```python
from build123d import *

# Parameters (mm, degrees)
CROQUIS1_W                 = 115
CROQUIS1_H                 = 76
SALIENTE_EXTRUIR1_DEPTH    = 1.5
CORTAR_EXTRUIR2_DEPTH      = 2.5
MATRIZL4_COUNT             = 3
MATRIZL4_PITCH             = 38.333333333
SIMETR_A1_COPY_1_DEPTH     = 2.5
SIMETR_A1_COPY_2_DEPTH     = 2.5
CORTAR_EXTRUIR3_DEPTH      = 2.5
MATRIZL5_COUNT             = 2
MATRIZL5_PITCH             = 38
SIMETR_A2_COPY_1_DEPTH     = 2.5
CROQUIS2_R                 = 1.2
CORTAR_EXTRUIR1_DEPTH      = 2.5
CORTAR_EXTRUIR1_DEPTH_BACK = 2.5
CROQUIS5_W                 = 9.5
CROQUIS5_H                 = 3
CROQUIS5_W_2               = 19
SALIENTE_EXTRUIR2_DEPTH    = 17
CROQUIS6_W                 = 19
CROQUIS6_H                 = 3
SALIENTE_EXTRUIR3_DEPTH    = 17


with BuildPart() as part:
    # Croquis1 → Saliente-Extruir1 (new body, symmetric)
    with BuildSketch(Plane(origin=(0, 0, 0), x_dir=(1, 0, 0), z_dir=(0, 1, 0))):
        Rectangle(CROQUIS1_W, CROQUIS1_H)
    extrude(amount=SALIENTE_EXTRUIR1_DEPTH, both=True)

    # Croquis3 → Cortar-Extruir2 (cut, symmetric)
    with BuildSketch(Plane(origin=(0, 0, 0), x_dir=(1, 0, 0), z_dir=(0, 1, 0))):
        Polygon((-47.916666667, -35), (-39.483333333, -35), (-37.183333333, -35), (-28.75, -35), (-28.75, -38), (-47.916666667, -38), align=None)
    cortar_extruir2 = extrude(amount=CORTAR_EXTRUIR2_DEPTH, both=True, mode=Mode.SUBTRACT)

    # MatrizL4: Cortar-Extruir2 ×3
    with Locations(*[(i * MATRIZL4_PITCH, 0, 0) for i in range(1, MATRIZL4_COUNT)]):
        add(cortar_extruir2, mode=Mode.SUBTRACT)

    # Simetría1: Cortar-Extruir2 across plane
    add(cortar_extruir2.mirror(Plane.XY), mode=Mode.SUBTRACT)

    # Simetría1 copy 1 sketch → Simetría1 copy 1 (cut, symmetric)
    with BuildSketch(Plane(origin=(38.333333333, 0, 0), x_dir=(1, 0, 0), z_dir=(0, 1, 0))):
        Polygon((-47.916666667, 35), (-39.483333333, 35), (-37.183333333, 35), (-28.75, 35), (-28.75, 38), (-47.916666667, 38), align=None)
    extrude(amount=SIMETR_A1_COPY_1_DEPTH, both=True, mode=Mode.SUBTRACT)

    # Simetría1 copy 2 sketch → Simetría1 copy 2 (cut, symmetric)
    with BuildSketch(Plane(origin=(76.666666667, 0, 0), x_dir=(1, 0, 0), z_dir=(0, 1, 0))):
        Polygon((-47.916666667, 35), (-39.483333333, 35), (-37.183333333, 35), (-28.75, 35), (-28.75, 38), (-47.916666667, 38), align=None)
    extrude(amount=SIMETR_A1_COPY_2_DEPTH, both=True, mode=Mode.SUBTRACT)

    # Croquis4 → Cortar-Extruir3 (cut, symmetric)
    with BuildSketch(Plane(origin=(0, 0, 0), x_dir=(1, 0, 0), z_dir=(0, 1, 0))):
        Polygon((-57.5, 28.5), (-54.5, 28.5), (-54.5, 20.15), (-54.5, 17.85), (-54.5, 9.5), (-57.5, 9.5), align=None)
    cortar_extruir3 = extrude(amount=CORTAR_EXTRUIR3_DEPTH, both=True, mode=Mode.SUBTRACT)

    # MatrizL5: Cortar-Extruir3 ×2
    with Locations(*[(0, 0, i * MATRIZL5_PITCH) for i in range(1, MATRIZL5_COUNT)]):
        add(cortar_extruir3, mode=Mode.SUBTRACT)

    # Simetría2: Cortar-Extruir3 across plane
    add(cortar_extruir3.mirror(Plane(origin=(0, 0, 0), x_dir=(0, 0, 1), z_dir=(1, 0, 0))), mode=Mode.SUBTRACT)

    # Simetría2 copy 1 sketch → Simetría2 copy 1 (cut, symmetric)
    with BuildSketch(Plane(origin=(0, 0, 38), x_dir=(-1, 0, 0), z_dir=(0, 1, 0))):
        Polygon((-57.5, -28.5), (-54.5, -28.5), (-54.5, -20.15), (-54.5, -17.85), (-54.5, -9.5), (-57.5, -9.5), align=None)
    extrude(amount=SIMETR_A2_COPY_1_DEPTH, both=True, mode=Mode.SUBTRACT)

    # Croquis2 → Cortar-Extruir1 (cut, two sides)
    with BuildSketch(Plane(origin=(0, 0, 0), x_dir=(1, 0, 0), z_dir=(0, 1, 0))) as cortar_extruir1_sk:
        with Locations((-50.22, 31.115)):
            Circle(CROQUIS2_R)
        with Locations((-50.22, -31.115)):
            Circle(CROQUIS2_R)
        with Locations((50.22, 31.115)):
            Circle(CROQUIS2_R)
        with Locations((50.22, -31.115)):
            Circle(CROQUIS2_R)
    extrude(amount=CORTAR_EXTRUIR1_DEPTH, mode=Mode.SUBTRACT)
    extrude(cortar_extruir1_sk.sketch, amount=-CORTAR_EXTRUIR1_DEPTH_BACK, mode=Mode.SUBTRACT)

    # Croquis5 → Saliente-Extruir2 (add)
    with BuildSketch(Plane.ZY.offset(57.5)):
        with Locations((-33.25, 0)):
            Rectangle(CROQUIS5_W, CROQUIS5_H)
        with Locations((33.25, 0)):
            Rectangle(CROQUIS5_W, CROQUIS5_H)
        Rectangle(CROQUIS5_W_2, CROQUIS5_H)
    extrude(amount=SALIENTE_EXTRUIR2_DEPTH)

    # Croquis6 → Saliente-Extruir3 (add)
    with BuildSketch(Plane.ZY.offset(54.5)):
        with Locations((19, 0)):
            Rectangle(CROQUIS6_W, CROQUIS6_H)
        with Locations((-19, 0)):
            Rectangle(CROQUIS6_W, CROQUIS6_H)
    extrude(amount=SALIENTE_EXTRUIR3_DEPTH)


solid = part.part
```
Design review of the part built by this model. Coordinates are the model's own, in mm. A direction names the side the tool comes from. Give positions to 0.01 mm unless a question says otherwise; leave off trailing zeros. Write each loop counter-clockwise with the first axis right and the second up, starting at its lowest first coordinate (ties: lowest second). Pieces come first, ordered by that corner, then holes. Notation, with made-up numbers: (4.25, 55.25) - (26.25, 55.25) arc R10 cw to (26.25, 64.25) - close; hole circle Ø9 at (42, 2.25). An arc over 180 degrees is marked (long way). Return JSON: item names as keys, results as strings. Group by question number.
(1) We need section A-A, the plane z = -26. Give the boundary of the cut face in (x, y), then the cut area to 3 significant figures.
(2) Insertion check: pin 1 (1.5 mm diameter, centred on y = 0, z = -14.5, fed in from +X); pin 2 (0.9 mm diameter, centred on y = 0.5, z = -15.5, fed in from -X); pin 3 (1.9 mm diameter, centred on x = -50.22, z = -31.115, fed in from +Y). Each pin has a flat end and moves straight along its axis. Give the tip position at first contact, or say it passes through.
(3) Mouldability with a two-part tool opening along Z and no side actions: class faces 4 (the flat face through (-19, 0, 38)), 5 (the flat face through (54.5, 0, -19)), 6 (the flat face through (56, 0, -9.5)), 7 (the flat face through (57.5, 0, 33)) as +Z half, -Z half, draft (parallel to the pull), parting line (faces both ways), or undercut.
(4) To check wall thickness, follow probe 1 along X at (y, z) = (0.8, -31); probe 2 along Z at (x, y) = (-50.22, 0.05) (3 decimals); probe 3 along X at (y, z) = (1.2, 20). State the ranges of each line that lie inside material, in increasing order.
(5) Machinability: for faces 1 (the flat face through (56, 0, -28.5)), 2 (the flat face through (38, 0, -35)), 3 (the flat face through (-47.917, 0, 37)), which of the approach directions +Z, -Z, +X, -X, +Y, -Y give a long, thin tool a straight path to every point of the face, cutting with its end or side? Answer none if there is none.
(6) We need section B-B, the plane y = -0.25. Give the number of separate pieces and of enclosed holes in the cut face, then the cut area to 3 significant figures.
Reported:
{
 "1": {"outline": "(-71.5, -1.5) - (54.5, -1.5) - (54.5, 1.5) - (-71.5, 1.5) - close", "area": "378 mm2"},
 "2": {"pin 1": "stops at x = 54.5", "pin 2": "stops at x = -71.5", "pin 3": "passes through"},
 "3": {"face 4": "+Z half", "face 5": "undercut", "face 6": "undercut", "face 7": "draft"},
 "4": {"probe 1": "x = -74.5 to -51.41, -49.03 to 49.03, 51.41 to 57.5", "probe 2": "z = -38 to -32.315, -29.915 to 29.915, 32.315 to 38", "probe 3": "x = -71.5 to 54.5"},
 "5": {"face 1": "+X, +Y, -Y", "face 2": "-Z, +Y, -Y", "face 3": "+Z, +Y, -Y"},
 "6": {"separate pieces": "1", "enclosed holes": "4", "area": "9,440 mm2"}
}
